Model file for the job. Use its own axes, mm. A direction names the side the tool comes from. Round coordinates to 2 decimals unless told otherwise and drop trailing zeros. Order: outer loops, then holes, each group sorted by start corner. A loop starts at its lowest first (then second) coordinate and runs counter-clockwise, first axis right, second up. Notation, with made-up numbers: (50, -23) -> (55, -23) arc R14 ccw to (55, -9) -> close; hole circle Ø6 at (-0.5, 5.5). An arc over 180 degrees is marked (long way). Put each result on its own line as item: value. Start each with the question number.
Q1. 3-axis set-ups, long thin cutter, end or side, ignore diameter. For faces 4 (the face through (2, -2, 0)), 5 (the face through (2.34, 0.6, 2.46)): which of +Z, -Z, +X, -X, +Y, -Y reach the whole face in a straight line?
Q2. Probe L1, parallel to Y at x = -0.75, z = 2.15; L2, parallel to X at y = 1.5, z = 4.6; L3, parallel to X at y = 0.25, z = 1.75. List the from-to ranges inside material, lowest first.
Q3. Cut at C-C, the plane x = 0.5. List the corners of the cut face in (y, z), and give its area (3 significant figures).
Q4. Pull direction X, two halves, no side cores. Call faces 1 (the face through (2, -2, 5)), 2 (the face through (-2.327, 0.646, 2.465)), 3 (the face through (-0.867, -3.905, 2.465)): released by +X, released by -X, zero draft, split by the parting line, or undercut.
Q5. Cut at A-A, the plane z = 4.4. List the corners of the cut face in (x, y), and give its area (3 significant figures).
Q6. Cut at D-D, the plane y = 2.75. List the corners of the cut face in (x, z), and give its area (3 significant figures).
Q7. Flat gauge pins, fed straight in: P1, Ø2, axis at y = 3, z = 1, coming from the -X side; P2, Ø2, axis at x = -0.5, z = 4, coming from the -Y side. Where does each tip first touch, or does it go through?
Q8. Cut at B-B, the plane y = 1.5. List the corners of the cut face in (x, z).
from build123d import *

# Parameters (mm, degrees)
F0_R     = 4
F1_DEPTH = 5


with BuildPart() as f1:
    # F0 (on Top) → F1 (new body)
    with BuildSketch(Plane.XY):
        Circle(F0_R)
        Polygon((-0.032408, -2.49979), (-1.277961, -2.148678), (-2.181086, -1.221829), (-2.49979, 0.032408), (-2.148678, 1.277961), (-1.221829, 2.181086), (0.032408, 2.49979), (1.277961, 2.148678), (2.181086, 1.221829), (2.49979, -0.032408), (2.148678, -1.277961), (1.221829, -2.181086), align=None, mode=Mode.SUBTRACT)
    extrude(amount=F1_DEPTH)


solid = f1.part
Ans:
1. face 4: -Z, +X, -X, +Y, -Y
1. face 5: +Z, -Z
2. L1: y = -3.93 to -2.3, 2.3 to 3.93
2. L2: x = -3.71 to -1.92, 1.91 to 3.71
2. L3: x = -3.99 to -2.44, 2.43 to 3.99
3. outline: (-3.97, 0) -> (-2.36, 0) -> (-2.36, 5) -> (-3.97, 5) -> close; (2.37, 0) -> (3.97, 0) -> (3.97, 5) -> (2.37, 5) -> close
3. area: 16.0 mm^2
4. face 1: zero draft
4. face 2: undercut
4. face 3: split by the parting line
5. outline: circle Ø8 at (0, 0); hole (-2.5, 0.03) -> (-2.18, -1.22) -> (-1.28, -2.15) -> (-0.03, -2.5) -> (1.22, -2.18) -> (2.15, -1.28) -> (2.5, -0.03) -> (2.18, 1.22) -> (1.28, 2.15) -> (0.03, 2.5) -> (-1.22, 2.18) -> (-2.15, 1.28) -> close
5. area: 31.5 mm^2
6. outline: (-2.9, 0) -> (2.9, 0) -> (2.9, 5) -> (-2.9, 5) -> close
6. area: 29.0 mm^2
7. P1: stops at x = -3.46
7. P2: stops at y = -4
8. outline: (-3.71, 0) -> (-1.92, 0) -> (-1.92, 5) -> (-3.71, 5) -> close; (1.91, 0) -> (3.71, 0) -> (3.71, 5) -> (1.91, 5) -> close
